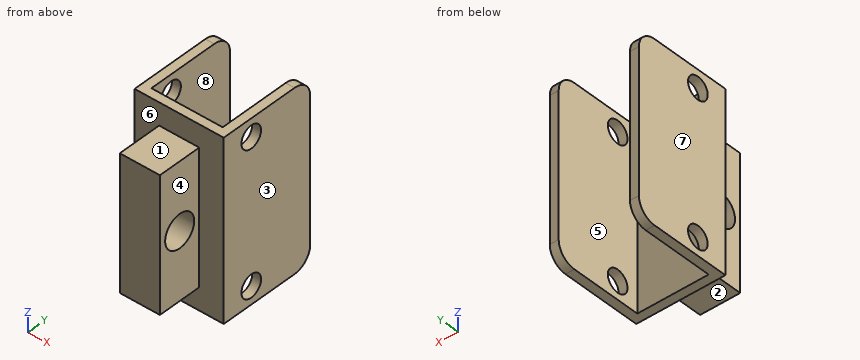
from build123d import *

# Parameters (mm, degrees)
EXTRUDE_THIN1_DEPTH = 50.8
FILLET1_R           = 5.08
SKETCH2_R           = 3.175
CUT_EXTRUDE1_DEPTH  = 63.217039467
SKETCH3_W           = 11.44
SKETCH3_H           = 38.1
BOSS_EXTRUDE1_DEPTH = 12.7
SKETCH4_R           = 4.699
CUT_EXTRUDE2_DEPTH  = 60.708428216


with BuildPart() as part:
    # Sketch1 → Extrude-Thin1 (new body)
    with BuildSketch(Plane.XY):
        Polygon((10.16, 25.4), (10.16, 0), (-10.16, 0), (-10.16, 25.4), (-12.7, 25.4), (-12.7, -2.54), (12.7, -2.54), (12.7, 25.4), align=None)
    extrude(amount=EXTRUDE_THIN1_DEPTH)

    # Fillet1
    fillet1_edges = [part.edges().sort_by_distance(p)[0] for p in [
        (-11.43, 25.4, 50.8),
        (-11.43, 25.4, 0),
        (11.43, 25.4, 50.8),
        (11.43, 25.4, 0),
    ]]
    fillet(fillet1_edges, radius=FILLET1_R)

    # Sketch2 → Cut-Extrude1 (cut, through all)
    with BuildSketch(Plane.ZY.offset(12.7)):
        with Locations((45.72, 6.35)):
            Circle(SKETCH2_R)
        with Locations((5.08, 6.35)):
            Circle(SKETCH2_R)
    extrude(amount=-CUT_EXTRUDE1_DEPTH, mode=Mode.SUBTRACT)

    # Sketch3 → Boss-Extrude1 (add)
    with BuildSketch(Plane.XZ.offset(2.54)):
        with Locations((0, 25.4)):
            Rectangle(SKETCH3_W, SKETCH3_H)
    extrude(amount=BOSS_EXTRUDE1_DEPTH)

    # Sketch4 → Cut-Extrude2 (cut, through all)
    with BuildSketch(Plane(origin=(5.72, 0, 0), x_dir=(0, 0, -1), z_dir=(1, 0, 0))):
        with Locations((-25.426069342, -8.852606466)):
            Circle(SKETCH4_R)
    extrude(amount=-CUT_EXTRUDE2_DEPTH, mode=Mode.SUBTRACT)


solid = part.part
The listing builds one solid part. Answer for the finished solid, in the listing's coordinates (mm). Face numbers are marked on the shaded views. A direction names the side the tool comes from. Give positions to 0.01 mm unless a question says otherwise; leave off trailing zeros. Order: outer loops, then holes, each group sorted by start corner. A loop starts at its lowest first (then second) coordinate and runs counter-clockwise, first axis right, second up. Notation, with made-up numbers: (20, -21) - (48, -21) arc R17 ccw to (48, -16) - close; hole circle Ø7 at (50, 12.25). An arc over 180 degrees is marked (long way). One line per item, written item: value. Start each with the question number.
1) A cutting plane is placed at B-B on y = 6.35. Give the vertices of the cut face in (x, z) (3 decimals).
2) A cutting plane is placed at C-C on z = 41. Give the vertices of the cut face in (x, y), then the cut area to 3 significant figures.
3) A tool of negligible diameter and unlimited length cuts with its end or side. For the marked faces 1, 2, 3, 4 and 5, from which of +Z, -Z, +X, -X, +Y, -Y can it reach the whole face along a straight path? Write none if from no direction.
4) A cutting plane is placed at D-D on x = -4. Give the vertices of the cut face in (y, z).
5) Find the intervals of material crossed by L1, parallel to Y at x = -11.6, z = 5.08 (3 decimals); L2, parallel to X at y = 19.5, z = 45.5; L3, parallel to Y at x = 3.25, z = 46, in increasing order.
6) A cutting plane is placed at A-A on x = 11. Give the vertices of the cut face in (y, z) (3 decimals).
7) The mould has two halves that part along X. Classify the marked faces 6, 7 and 8: released by +X, released by -X, zero draft, split by the parting line, or undercut.
8) Given pin 1 Ø4 at (x, z) = (4.5, 7) entering from +Y; pin 2 Ø9 at (x, y) = (-1, -9) entering from +Z; pin 3 Ø9 at (x, y) = (0, -9) entering from -Z, each flat-ended and moving along its own axis, determine where each tip first touches the part or whether it passes through.
Answer sheet:
1. outline: (-12.7, 0) - (-10.16, 0) - (-10.16, 1.905) - (-12.7, 1.905) - close; (-12.7, 8.255) - (-10.16, 8.255) - (-10.16, 42.545) - (-12.7, 42.545) - close; (-12.7, 48.895) - (-10.16, 48.895) - (-10.16, 50.8) - (-12.7, 50.8) - close; (10.16, 0) - (12.7, 0) - (12.7, 1.905) - (10.16, 1.905) - close; (10.16, 8.255) - (12.7, 8.255) - (12.7, 42.545) - (10.16, 42.545) - close; (10.16, 48.895) - (12.7, 48.895) - (12.7, 50.8) - (10.16, 50.8) - close
2. outline: (-12.7, -2.54) - (-5.72, -2.54) - (-5.72, -15.24) - (5.72, -15.24) - (5.72, -2.54) - (12.7, -2.54) - (12.7, 25.4) - (10.16, 25.4) - (10.16, 0) - (-10.16, 0) - (-10.16, 25.4) - (-12.7, 25.4) - close
2. area: 339 mm2
3. face 1: +Z, +X, -X, -Y
3. face 2: -Z, +X, -X, -Y
3. face 3: +Z, -Z, +X, +Y, -Y
3. face 4: +Z, -Z, +X, -Y
3. face 5: +Z, -Z, +Y
4. outline: (-15.24, 6.35) - (-2.54, 6.35) - (-2.54, 0) - (0, 0) - (0, 50.8) - (-2.54, 50.8) - (-2.54, 44.45) - (-15.24, 44.45) - close; hole circle Ø9.4 at (-8.85, 25.43)
5. L1: y = -2.54 to 3.175, 9.525 to 25.4
5. L2: x = -12.7 to -10.16, 10.16 to 12.7
5. L3: y = -2.54 to 0
6. outline: (-2.54, 0) - (20.32, 0) arc R5.08 ccw to (25.4, 5.08) - (25.4, 45.72) arc R5.08 ccw to (20.32, 50.8) - (-2.54, 50.8) - close; hole circle Ø6.35 at (6.35, 5.08); hole circle Ø6.35 at (6.35, 45.72)
7. face 6: zero draft
7. face 7: released by -X
7. face 8: undercut
8. pin 1: stops at y = 0
8. pin 2: stops at z = 44.45
8. pin 3: stops at z = 6.35
